Check sheet for the drawn part. Datum: minimum x, y, z corner. Units: mm. Coordinates: 2 decimals unless noted, no trailing zeros. Order: outer loops, then holes, each group sorted by start corner. A loop starts at its lowest first (then second) coordinate and runs counter-clockwise, first axis right, second up. Notation, with made-up numbers: (-36, 10) - (10, 10) arc R9 ccw to (10, 21) - close; hole circle Ø6 at (17, 40.25). An arc over 180 degrees is marked (long way). One line per item, written item: value. Start each with the question number.
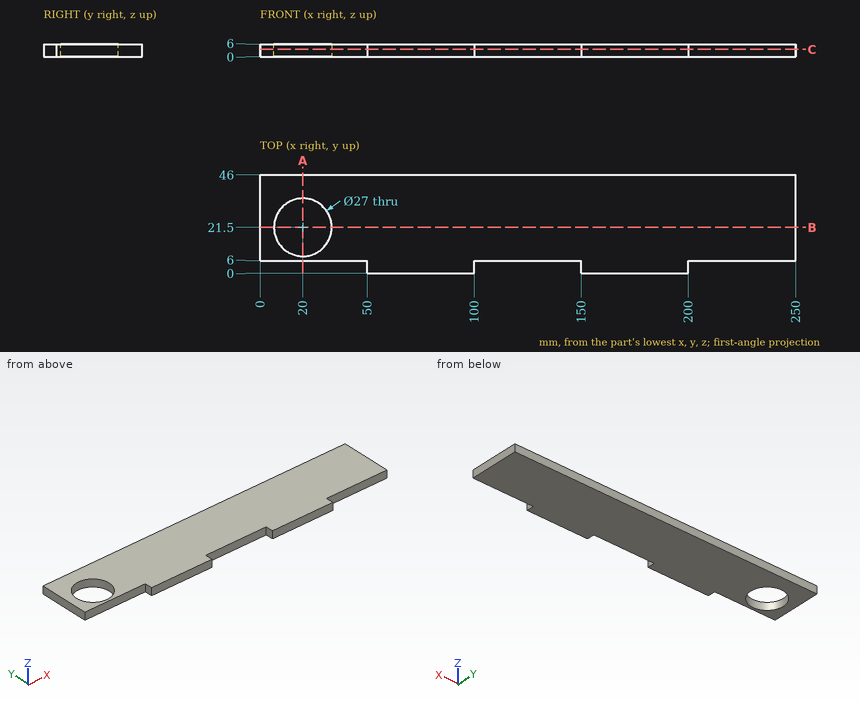
Q1. Material ranges on probe 1 along Y at (x, z) = (20, 4.2); probe 2 along X at (y, z) = (20.5, 5.45); probe 3 along X at (y, z) = (14, 4.5), recorded low to high.
Q2. Cross-section at B-B, the plane y = 21.5. Enter the section's corners in (x, z).
Q3. Gauge pin test, flat ends, axial feed: P1, Ø1.8, axis at y = 2.5, z = 2, coming from the -X side; P2, Ø1.8, axis at y = 2, z = 3.5, coming from the +X side; P3, Ø1, axis at x = 134.5, z = 0.5, coming from the -Y side. Record the tip position at first contact, or that the pin passes through.
Q4. Cross-section at A-A, the plane x = 20. Enter the section's corners in (y, z), and give its area (3 significant figures).
Q5. Cross-section at C-C, the plane z = 3.5. Enter the section's corners in (x, y), and give its area (3 significant figures).
Check result:
1. probe 1: y = 6 to 8, 35 to 46
1. probe 2: x = 0 to 6.54, 33.46 to 250
1. probe 3: x = 0 to 8.78, 31.22 to 250
2. outline: (0, 0) - (6.5, 0) - (6.5, 6) - (0, 6) - close; (33.5, 0) - (250, 0) - (250, 6) - (33.5, 6) - close
3. P1: stops at x = 50
3. P2: stops at x = 200
3. P3: stops at y = 6
4. outline: (6, 0) - (8, 0) - (8, 6) - (6, 6) - close; (35, 0) - (46, 0) - (46, 6) - (35, 6) - close
4. area: 78.0 mm2
5. outline: (0, 6) - (50, 6) - (50, 0) - (100, 0) - (100, 6) - (150, 6) - (150, 0) - (200, 0) - (200, 6) - (250, 6) - (250, 46) - (0, 46) - close; hole circle Ø27 at (20, 21.5)
5. area: 10,000 mm2
